```python
from build123d import *

# Parameters (mm, degrees)
BOSS_EXTRUDE2_DEPTH = 50.8
SKETCH2_R           = 3.96875
SKETCH2_R_2         = 2.75
BOSS_EXTRUDE3_DEPTH = 12.7
SKETCH3_R           = 3.96875
SKETCH3_R_2         = 2.75
BOSS_EXTRUDE4_DEPTH = 12.7


with BuildPart() as part:
    # Sketch1 → Boss-Extrude2 (new body)
    with BuildSketch(Plane(origin=(0, 0, 0), x_dir=(1, 0, 0), z_dir=(0, 1, 0))):
        with BuildLine():
            Line((14.199031657, 12.7), (-14.199031657, 12.7))
            ThreePointArc((-14.199031657, 12.7), (-19.05, 0), (-14.199031657, -12.7))
            Line((-14.199031657, -12.7), (14.199031657, -12.7))
            ThreePointArc((14.199031657, -12.7), (17.795983438, -6.79746081), (19.05, 0))
            ThreePointArc((19.05, 0), (17.795983438, 6.79746081), (14.199031657, 12.7))
        make_face()
    extrude(amount=BOSS_EXTRUDE2_DEPTH)

    # Sketch2 → Boss-Extrude3 (add)
    with BuildSketch(Plane(origin=(0, 50.8, 0), x_dir=(1, 0, 0), z_dir=(0, 1, 0))):
        with Locations((3.96875, 0)):
            Circle(SKETCH2_R)
        with Locations((3.96875, 0)):
            Circle(SKETCH2_R_2, mode=Mode.SUBTRACT)
    extrude(amount=BOSS_EXTRUDE3_DEPTH)

    # Sketch3 → Boss-Extrude4 (add)
    with BuildSketch(Plane(origin=(0, 0, -12.7), x_dir=(-1, 0, 0), z_dir=(0, 0, -1))):
        with Locations((3.96875, 44.83125)):
            Circle(SKETCH3_R)
        with Locations((3.96875, 44.83125)):
            Circle(SKETCH3_R_2, mode=Mode.SUBTRACT)
    extrude(amount=BOSS_EXTRUDE4_DEPTH)


solid = part.part
```
For this review, take the finished solid that the model builds, in its own axes (mm). A direction names the side the tool comes from. Give positions to 0.01 mm unless a question says otherwise; leave off trailing zeros. Loops run counter-clockwise (first coordinate to the right, second up) from the corner with the lowest first, then second, coordinate; pieces in that order, holes last. Notation, with made-up numbers: M -18.75,-14.75 L 3.25,-14.75 A18 cw 3.25,6.25 Z; hole C -13.75,29 d11. An arc over 180 degrees is marked long. One line per item, written item: value. Start each with the question number.
Q1. Clearance check with flat-ended pins moving along their axes: pin 1 Ø4.5 at (x, y) = (-3.97, 44.83) entering from -Z; pin 2 Ø6 at (y, z) = (26.5, -16) entering from -X. State where each tip first meets the part, or that it passes through.
Q2. Add section C-C (y = 22.5). Give the boundary of the cut face in (x, z).
Q3. Add section D-D (z = -19). Give the boundary of the cut face in (x, y), and give its area (3 significant figures).
Q4. Draft analysis for pull direction X (two halves, no side actions). For faces 1 (the face through (-3, 42, -25.4)), 2 (the face through (4, 50.8, 0)), 3 (the face through (-3.108, 40.957, -18.961)), 4 (the face through (-19.05, 25.04, -0.19)), state which applies: released by +X, released by -X, zero draft, split by the parting line, or undercut.
Q5. Add section B-B (z = -1). Give the boundary of the cut face in (x, y), and give its area (3 significant figures).
Q6. Add section A-A (x = -9.5). Give the boundary of the cut face in (y, z), and give its area (3 significant figures).
Q7. For L1, parallel to X at y = 58, z = 0; L2, parallel to Z at x = 3, y = 44; L3, parallel to Y at x = 0, z = -2.5, list the stretches that pass through material, from the lowest coordinate up.
Q8. Machinability: for faces 5 (the face through (7.754, 57.061, -1.192)), 6 (the face through (-4, 45, -12.7)), 7 (the face through (0, 25, 12.7)), which of the approach directions +Z, -Z, +X, -X, +Y, -Y give a long, thin tool a straight path to every point of the face, cutting with its end or side? Answer none if there is none.
Reply:
1. pin 1: z = -12.7
1. pin 2: through
2. outline: M -14.2,-12.7 L 14.2,-12.7 A19.05 ccw 14.2,12.7 L -14.2,12.7 A19.05 ccw Z
3. outline: C -3.97,44.83 d7.94; hole C -3.97,44.83 d5.5
3. area: 25.7 mm²
4. face 1: zero draft
4. face 2: undercut
4. face 3: split by the parting line
4. face 4: released by -X
5. outline: M -19.02,0 L 19.02,0 L 19.02,50.8 L 7.81,50.8 L 7.81,63.5 L 6.53,63.5 L 6.53,50.8 L 1.41,50.8 L 1.41,63.5 L 0.13,63.5 L 0.13,50.8 L -19.02,50.8 Z
5. area: 1,970 mm²
6. outline: M 0,-12.7 L 50.8,-12.7 L 50.8,12.7 L 0,12.7 Z
6. area: 1,290 mm²
7. L1: 0 to 1.22, 6.72 to 7.94
7. L2: -12.7 to 12.7
7. L3: 0 to 50.8
8. face 5: +Y
8. face 6: -Z
8. face 7: +Z, +X, -X, +Y, -Y
